Geometry check sheet. Reference: the model listing, model coordinates, mm. Face numbers are marked on the shaded views. A direction names the side the tool comes from. Give positions to 0.01 mm unless a question says otherwise; leave off trailing zeros. Loops run counter-clockwise (first coordinate to the right, second up) from the corner with the lowest first, then second, coordinate; pieces in that order, holes last. Notation, with made-up numbers: (14, 72) -> (23, 72) arc R13 ccw to (23, 88) -> close; hole circle Ø11 at (-14.5, -25.75). An arc over 180 degrees is marked (long way). Write item = value, one per line. Start each with the question number.
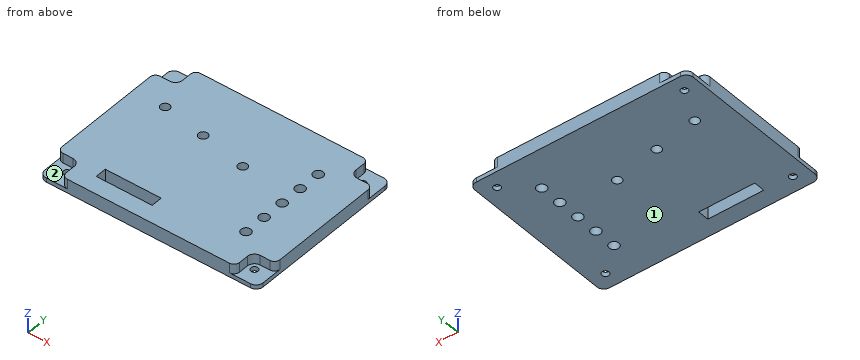
```python
from build123d import *

# Parameters (mm, degrees)
SKETCH1_R           = 3.25
SKETCH1_R_2         = 3.5
SKETCH1_W           = 40
SKETCH1_H           = 8
BOSS_EXTRUDE1_DEPTH = 10
CUT_EXTRUDE1_DEPTH  = 7
SKETCH3_R           = 2.5
CUT_EXTRUDE2_DEPTH  = 10
FILLET1_R           = 4


with BuildPart() as part:
    # Sketch1 → Boss-Extrude1 (new body)
    with BuildSketch(Plane.XY):
        with BuildLine():
            Line((-67.614699332, 37.697104677), (78.385300668, 37.697104677))
            ThreePointArc((78.385300668, 37.697104677), (81.920834574, 36.232638583), (83.385300668, 32.697104677))
            Line((83.385300668, 32.697104677), (83.385300668, -75.302895323))
            ThreePointArc((83.385300668, -75.302895323), (81.920834574, -78.838429229), (78.385300668, -80.302895323))
            Line((78.385300668, -80.302895323), (-67.614699332, -80.302895323))
            ThreePointArc((-67.614699332, -80.302895323), (-71.150233238, -78.838429229), (-72.614699332, -75.302895323))
            Line((-72.614699332, -75.302895323), (-72.614699332, 32.697104677))
            ThreePointArc((-72.614699332, 32.697104677), (-71.150233238, 36.232638583), (-67.614699332, 37.697104677))
        make_face()
        with Locations((-49.614699332, 2.697104677)):
            Circle(SKETCH1_R, mode=Mode.SUBTRACT)
        with Locations((-17.614699332, -3.302895323)):
            Circle(SKETCH1_R, mode=Mode.SUBTRACT)
        with Locations((16.385300668, -10.302895323)):
            Circle(SKETCH1_R, mode=Mode.SUBTRACT)
        with Locations((53.385300668, 10.697104677)):
            Circle(SKETCH1_R_2, mode=Mode.SUBTRACT)
        with Locations((53.385300668, -5.302895323)):
            Circle(SKETCH1_R_2, mode=Mode.SUBTRACT)
        with Locations((53.385300668, -21.302895323)):
            Circle(SKETCH1_R_2, mode=Mode.SUBTRACT)
        with Locations((53.385300668, -37.302895323)):
            Circle(SKETCH1_R_2, mode=Mode.SUBTRACT)
        with Locations((53.385300668, -53.302895323)):
            Circle(SKETCH1_R_2, mode=Mode.SUBTRACT)
        with Locations((-21.614699332, -64.302895323)):
            Rectangle(SKETCH1_W, SKETCH1_H, mode=Mode.SUBTRACT)
    extrude(amount=BOSS_EXTRUDE1_DEPTH)

    # Sketch2 → Cut-Extrude1 (cut)
    with BuildSketch(Plane.XY.offset(10)):
        with BuildLine():
            Line((-72.614699332, 37.697104677), (-56.614699332, 37.697104677))
            Line((-56.614699332, 37.697104677), (-56.614699332, 26.697104677))
            ThreePointArc((-56.614699332, 26.697104677), (-58.079165426, 23.161570771), (-61.614699332, 21.697104677))
            Line((-61.614699332, 21.697104677), (-72.614699332, 21.697104677))
            Line((-72.614699332, 21.697104677), (-72.614699332, 37.697104677))
        make_face()
        with BuildLine():
            Line((83.385300668, 37.697104677), (67.385300668, 37.697104677))
            Line((67.385300668, 37.697104677), (67.385300668, 26.697104677))
            ThreePointArc((67.385300668, 26.697104677), (68.849766762, 23.161570771), (72.385300668, 21.697104677))
            Line((72.385300668, 21.697104677), (83.385300668, 21.697104677))
            Line((83.385300668, 21.697104677), (83.385300668, 37.697104677))
        make_face()
        with BuildLine():
            Line((83.385300668, -80.302895323), (67.385300668, -80.302895323))
            Line((67.385300668, -80.302895323), (67.385300668, -69.302895323))
            ThreePointArc((67.385300668, -69.302895323), (68.849766762, -65.767361417), (72.385300668, -64.302895323))
            Line((72.385300668, -64.302895323), (83.385300668, -64.302895323))
            Line((83.385300668, -64.302895323), (83.385300668, -80.302895323))
        make_face()
        with BuildLine():
            Line((-72.614699332, -80.302895323), (-56.614699332, -80.302895323))
            Line((-56.614699332, -80.302895323), (-56.614699332, -69.302895323))
            ThreePointArc((-56.614699332, -69.302895323), (-58.079165426, -65.767361417), (-61.614699332, -64.302895323))
            Line((-61.614699332, -64.302895323), (-72.614699332, -64.302895323))
            Line((-72.614699332, -64.302895323), (-72.614699332, -80.302895323))
        make_face()
    extrude(amount=-CUT_EXTRUDE1_DEPTH, mode=Mode.SUBTRACT)

    # Sketch3 → Cut-Extrude2 (cut)
    with BuildSketch(Plane.XY.offset(3)):
        with Locations((-61.614699332, 26.697104677)):
            Circle(SKETCH3_R)
        with Locations((72.385300668, 26.697104677)):
            Circle(SKETCH3_R)
        with Locations((72.385300668, -69.302895323)):
            Circle(SKETCH3_R)
        with Locations((-61.614699332, -69.302895323)):
            Circle(SKETCH3_R)
    extrude(amount=-CUT_EXTRUDE2_DEPTH, mode=Mode.SUBTRACT)

    # Fillet1
    fillet1_edges = [part.edges().sort_by_distance(p)[0] for p in [
        (83.385300668, -64.302895323, 6.5),
        (67.385300668, -80.302895323, 6.5),
        (67.385300668, 37.697104677, 6.5),
        (83.385300668, 21.697104677, 6.5),
        (-72.614699332, 21.697104677, 6.5),
        (-56.614699332, 37.697104677, 6.5),
        (-56.614699332, -80.302895323, 6.5),
        (-72.614699332, -64.302895323, 6.5),
    ]]
    fillet(fillet1_edges, radius=FILLET1_R)


solid = part.part
```
1) Thickness scan on line 1 (Y direction, x = -4.5, z = 3.5); line 2 (X direction, y = 11, z = 4.5); line 3 (X direction, y = -22, z = 4.75). Record the ranges inside material, lowest first.
2) Depth check by flat-ended pin: pin 1 Ø1.5 at (x, z) = (65, 4.5) entering from -Y; pin 2 Ø1.5 at (x, y) = (9.5, -41) entering from -Z; pin 3 Ø10 at (x, y) = (-66.5, -72) entering from +Z; pin 4 Ø5.5 at (x, z) = (76.5, 6) entering from -Y. Enter the tip coordinate at first touch or a pass-through.
3) Section check A-A (y = -19.5). Enter the section's corners in (x, z).
4) Section check B-B (z = 1.5). Give the number of separate pieces and of enclosed holes in the cut face, plus the area to 3 significant figures.
5) Tool access check on the marked faces 1 and 2. Record the directions out of +Z, -Z, +X, -X, +Y, -Y that give a thin tool (end or side, any length) a straight path to the whole face; none if there is none.
Check result:
q1.line_1 = -80.3 to -68.3, -60.3 to 37.7
q1.line_2 = -72.61 to 49.9, 56.87 to 83.39
q1.line_3 = -72.61 to 49.96, 56.82 to 83.39
q2.pin_1 = -80.21
q2.pin_2 = 0
q2.pin_3 = 3
q2.pin_4 = -64.3
q3.outline = (-72.61, 0) -> (50.39, 0) -> (50.39, 10) -> (-72.61, 10) -> close; (56.39, 0) -> (83.39, 0) -> (83.39, 10) -> (56.39, 10) -> close
q4.separate_pieces = 1
q4.enclosed_holes = 13
q4.area = 17,700 mm2
q5.face_1 = -Z, +X, -X, +Y, -Y
q5.face_2 = +Z, -X, -Y
